For this review, take the finished solid that the model builds, in its own axes (mm). A direction names the side the tool comes from. Coordinates: 2 decimals unless noted, no trailing zeros. Write each loop counter-clockwise with the first axis right and the second up, starting at its lowest first coordinate (ties: lowest second). Pieces come first, ordered by that corner, then holes.
1) We need section D-D on y = 5.25. Write out the cut boundary in (x, z), then the cut area to 3 significant figures.
2) We need section B-B on z = 0. Write out the cut boundary in (x, y), then the cut area to 3 significant figures.
3) For faces 1 (the face through (8.6, 0.7, -7.8)), 2 (the face through (-9, 7.955, 6)), 3 (the face through (-10.485, 2.448, 4.347)), list the 3-axis set-ups (+Z, -Z, +X, -X, +Y, -Y) from which the entire face can be reached by the end or side of a thin tool; tool diameter is ignored.
4) We need section A-A on x = 0. Write out the cut boundary in (y, z).
5) We need section C-C on y = 1. Write out the cut boundary in (x, z), then the cut area to 3 significant figures.
6) Insertion check: P1, Ø12, axis at x = 0, z = 0, coming from the +Y side; P2, Ø2, axis at x = -9.5, y = 5, coming from the -Z side; P3, Ø2, axis at y = 5.5, z = 7.5, coming from the -X side; P4, Ø4, axis at y = 3, z = -7.5, coming from the +X side. Each pin has a flat end and moves straight along its axis. Give the tip position at first contact, or say it passes through.
7) Mouldability with a two-part tool opening along Z and no side actions: class faces 4 (the face through (-5.86, 5.42, 11.267)), 5 (the face through (8.05, 3.76, 6.18)), 6 (the face through (0.1, -0.545, 10.3)) as pulls with the +Z half, pulls with the -Z half, needs draft (parallel to the pull), parting line crosses it, or undercut.
8) To check wall thickness, follow line 1 along Z through (x, y) = (0, 2.75); line 2 along Y through (x, z) = (11.25, 2); line 3 along Z through (x, y) = (0, 6.25). State the ranges of each line that lie inside material, in increasing order.
from build123d import *


with BuildPart() as part:
    # 草图1 → 旋转1 (revolve)
    with BuildSketch(Plane.XY, mode=Mode.PRIVATE) as revolve_1_sk:
        Polygon((10.15, -0.545464411), (10.15, 7.954535589), (12.7, 7.954535589), (12.7, 2.954535589), (11.35, 2.954535589), (11.35, 1.954535589), (11.61, 1.954535589), (11.61, -0.545464411), align=None)
    revolve(revolve_1_sk.sketch.rotate(Axis((0, 16.886018237, 0), (0, -1, 0)), 180), axis=Axis((0, 16.886018237, 0), (0, -1, 0)))  # turned: the seam where the file's is


solid = part.part
Result:
1. outline: circle Ø25.4 at (0, 0); hole circle Ø20.3 at (0, 0)
1. area: 183 mm2
2. outline: (-12.7, 2.95) - (-11.35, 2.95) - (-11.35, 1.95) - (-11.61, 1.95) - (-11.61, -0.55) - (-10.15, -0.55) - (-10.15, 7.95) - (-12.7, 7.95) - close; (10.15, -0.55) - (11.61, -0.55) - (11.61, 1.95) - (11.35, 1.95) - (11.35, 2.95) - (12.7, 2.95) - (12.7, 7.95) - (10.15, 7.95) - close
2. area: 35.2 mm2
3. face 1: -Y
3. face 2: +Z, -Z, +X, -X, +Y
3. face 3: none
4. outline: (-0.55, -11.61) - (1.95, -11.61) - (1.95, -11.35) - (2.95, -11.35) - (2.95, -12.7) - (7.95, -12.7) - (7.95, -10.15) - (-0.55, -10.15) - close; (-0.55, 10.15) - (7.95, 10.15) - (7.95, 12.7) - (2.95, 12.7) - (2.95, 11.35) - (1.95, 11.35) - (1.95, 11.61) - (-0.55, 11.61) - close
5. outline: circle Ø23.22 at (0, 0); hole circle Ø20.3 at (0, 0)
5. area: 99.8 mm2
6. P1: passes through
6. P2: stops at z = -9.44
6. P3: stops at x = -10.91
6. P4: stops at x = 11.45
7. face 4: parting line crosses it
7. face 5: undercut
7. face 6: needs draft
8. line 1: z = -11.35 to -10.15, 10.15 to 11.35
8. line 2: y = -0.55 to 1.95, 2.95 to 7.95
8. line 3: z = -12.7 to -10.15, 10.15 to 12.7
